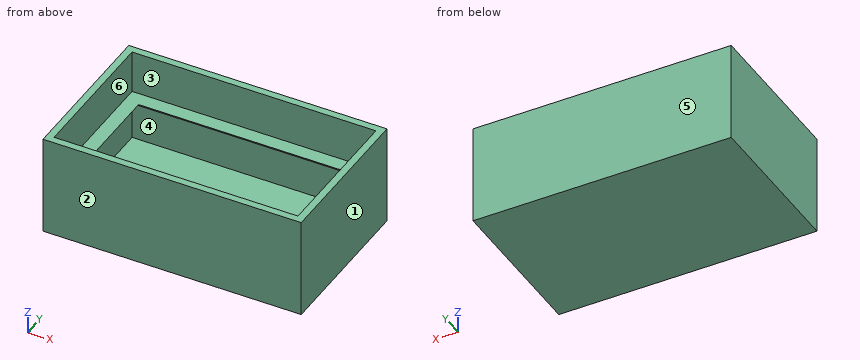
from build123d import *

# Parameters (mm, degrees)
F1_W     = 180
F1_H     = 110
F1_W_2   = 170
F1_H_2   = 100
F2_DEPTH = 70
F0_W     = 180
F0_H     = 110
F3_DEPTH = 5
F5_W     = 170
F5_H     = 100
F5_W_2   = 160
F5_H_2   = 90
F6_DEPTH = 5
F6_TAPER = -45


with BuildPart() as f2:
    # F1 (on face) → F2 (new body)
    with BuildSketch(Plane.XY):
        Rectangle(F1_W, F1_H)
        Rectangle(F1_W_2, F1_H_2, mode=Mode.SUBTRACT)
    extrude(amount=F2_DEPTH)

    # F0 (on Top) → F3 (join)
    with BuildSketch(Plane.XY):
        Rectangle(F0_W, F0_H)
    extrude(amount=F3_DEPTH)

    # F5 (on offset) → F6 (join)
    with BuildSketch(Plane.XY.offset(35)):
        Rectangle(F5_W, F5_H)
        Rectangle(F5_W_2, F5_H_2, mode=Mode.SUBTRACT)
    extrude(amount=F6_DEPTH, taper=F6_TAPER)


solid = f2.part
Geometry: final body of the model. Coordinates: model frame, mm. Face numbers are marked on the shaded views. A direction names the side the tool comes from. Round coordinates to 2 decimals unless told otherwise and drop trailing zeros. Loops run counter-clockwise (first coordinate to the right, second up) from the corner with the lowest first, then second, coordinate; pieces in that order, holes last.
Q1. Section A-A on z = 15.5. Return loops of the section in (x, y).
Q2. Material intervals for L1, parallel to X at y = 37.5, z = 10; L2, parallel to Y at x = -41, z = 28.5; L3, parallel to Z at x = 22.5, y = 36, sorted ascending.
Q3. Pull-direction query (X, two-part tool) for the marked faces 1, 2 and 3; classes: released by +X, released by -X, zero draft, split by the parting line, or undercut.
Q4. Access query for the marked faces 4, 5 and 6. Directions: +Z, -Z, +X, -X, +Y, -Y. A direction counts if a zero-diameter tool reaches every point of the face in a straight line with its end or side. Return the directions, or none.
Evaluation:
1. outline: (-90, -55) - (90, -55) - (90, 55) - (-90, 55) - close; hole (-85, -50) - (85, -50) - (85, 50) - (-85, 50) - close
2. L1: x = -90 to -85, 85 to 90
2. L2: y = -55 to -50, 50 to 55
2. L3: z = 0 to 5
3. face 1: released by +X
3. face 2: zero draft
3. face 3: undercut
4. face 4: none
4. face 5: +Z, -Z, +X, -X, +Y
4. face 6: +Z
